```python
from build123d import *

# Parameters (mm, degrees)
F1_DEPTH = 7


with BuildPart() as f1:
    # F0 (on Front) → F1 (new body)
    with BuildSketch(Plane.XZ):
        with BuildLine():
            ThreePointArc((-18.6193257059, 24.4526938776), (-17.4724085616, 23.0101324022), (-17.0632034356, 21.2132034356))
            ThreePointArc((-17.0632034356, 21.2132034356), (-18.2107776829, 18.3482532441), (-21.0188369777, 17.0677575392))
            Line((-21.0188369777, 17.0677575392), (-22.249362675, 13.2805888584))
            ThreePointArc((-22.249362675, 13.2805888584), (-15.3241365798, 15.7985112404), (-13.3952950657, 22.9103506653))
            Line((-13.3952950657, 22.9103506653), (-13.4874691837, 25.2643290081))
            Line((-13.4874691837, 25.2643290081), (-18.3556094659, 25.2643290081))
            Line((-18.3556094659, 25.2643290081), (-18.6193257059, 24.4526938776))
        make_face()
    extrude(amount=F1_DEPTH)


solid = f1.part
```
Design review of the part built by this model. Coordinates are the model's own, in mm. Give positions to 0.01 mm unless a question says otherwise; leave off trailing zeros. Order: outer loops, then holes, each group sorted by start corner. A loop starts at its lowest first (then second) coordinate and runs counter-clockwise, first axis right, second up. Notation, with made-up numbers: (8, 88.5) -> (21, 88.5) arc R22 ccw to (21, 106.5) -> close; hole circle Ø9 at (-1, -6.75). An arc over 180 degrees is marked (long way). Write item = value, one per line. Start each with the question number.
(1) We need section D-D on x = -14.75. Write out the cut boundary in (y, z), plus the area to 3 significant figures.
(2) We need section C-C on z = 17.5. Write out the cut boundary in (x, y).
(3) We need section A-A on y = -0.5. Write out the cut boundary in (x, z).
(4) We need section B-B on x = -18. Write out the cut boundary in (y, z).
(5) To check wall thickness, follow line 1 along X through (y, z) = (-5.5, 21.25); line 2 along Z through (x, y) = (-17.5, -4); line 3 along Z through (x, y) = (-18.25, -1.5). State the ranges of each line that lie inside material, in increasing order.
(6) For pin 1 (1 mm diameter, centred on y = -1, z = 17, fed in from -X); pin 2 (4 mm diameter, centred on y = -2.5, z = 17, fed in from -X); pin 3 (3 mm diameter, centred on y = -6, z = 20, fed in from +X); pin 4 (1.5 mm diameter, centred on x = -19, z = 20.5, fed in from +Y), all flat-tipped, find the tip position at first contact; note any pin that passes through.
Numbers:
q1.outline = (-7, 16.5) -> (0, 16.5) -> (0, 25.26) -> (-7, 25.26) -> close
q1.area = 61.4 mm^2
q2.outline = (-19.36, -7) -> (-14.13, -7) -> (-14.13, 0) -> (-19.36, 0) -> close
q3.outline = (-22.25, 13.28) arc R8 ccw to (-13.4, 22.91) -> (-13.49, 25.26) -> (-18.36, 25.26) -> (-18.62, 24.45) arc R4.15 cw to (-21.02, 17.07) -> close
q4.outline = (-7, 13.89) -> (0, 13.89) -> (0, 18.59) -> (-7, 18.59) -> close; (-7, 23.84) -> (0, 23.84) -> (0, 25.26) -> (-7, 25.26) -> close
q5.line_1 = -17.06 to -13.21
q5.line_2 = 14.13 to 19.36, 23.07 to 25.26
q5.line_3 = 13.78 to 18.31, 24.12 to 25.26
q6.pin_1 = -21.2
q6.pin_2 = -21.69
q6.pin_3 = -13.21
q6.pin_4 = through
